Autodesk Inventor part; units mm, degrees
ref_plane "YZ Plane" through (0, 0, 0) normal (1, 0, 0) x (0, 1, 0)
ref_plane "XY Plane" through (0, 0, 0) normal (0, 0, 1) x (1, 0, 0)
sketch "Sketch1" plane through (0, 0, 0) normal (0, 1, 0) x (-1, 0, 0)
  circle A0 centre (0, 0) radius 101.6
  dimension "d0" = 203.2
extrude "Extrusion1" add sketch "Sketch1" along normal mid plane 9.525
sketch "Sketch2" plane through (0, 4.7625, 0) normal (0, 1, 0) x (1, 0, 0)
  circle A0 centre (0, 0) radius 111.125
  dimension "d3" = 222.25
extrude "Extrusion2" add sketch "Sketch2" along normal blind 6.35
mirror "Mirror1" about plane through (0, 0, 0) normal (0, 1, 0) of "Extrusion2"
sketch "Sketch4" plane through (0, 11.1125, 0) normal (0, 1, 0) x (1, 0, 0)
  circle A0 centre (0, 23.8125) radius 2.54
  circle A1 centre (-20.6222, 11.9063) radius 2.54
  circle A2 centre (-20.6222, -11.9062) radius 2.54
  circle A3 centre (0, -23.8125) radius 2.54
  circle A4 centre (20.6222, -11.9063) radius 2.54
  circle A5 centre (20.6222, 11.9062) radius 2.54
  point P0 (0, 0)
  dimension "d6" = 5.08
  dimension "d7" = 23.8125
  dimension "d10" = 360
extrude "Extrusion3" cut sketch "Sketch4" against normal through all
sketch "Sketch5" plane through (0, 11.1125, 0) normal (0, 1, 0) x (1, 0, 0)
  circle A0 centre (0, 0) radius 5
  dimension "d14" = 10
extrude "Extrusion4" cut sketch "Sketch5" against normal through all
equation "\"d0\" = innerDiam"
equation "\"d1\" = innerWidth"
equation "\"d3\" = outerDiam"
equation "\"d4\" = outerWidth"
equation "\"d12\" = outerWidth"
equation "\"d15\" = outerWidth"
equation "\"innerDiam\" = 203.2"
equation "\"innerRadius\" = 0.5 * innerDiam"
equation "\"outerDiam\" = 2 * outerRadius"
equation "\"innerWidth\" = 9.525"
equation "\"outerWidth\" = 6.35"
properties part number "WoodPully"
Build history of the part. All positions in model axes, mm. A direction names the side the tool comes from. Round coordinates to 2 decimals unless told otherwise and drop trailing zeros. Write each loop counter-clockwise with the first axis right and the second up, starting at its lowest first coordinate (ties: lowest second). Pieces come first, ordered by that corner, then holes.
1) Band-saw the part on B-B, the plane x = 0. List the corners of the cut face in (y, z) (1 decimal).
2) 3-axis set-ups, long thin cutter, end or side, ignore diameter. For faces 5 (the flat face through (49, 4.762, 90)), 6 (the flat face through (23, 11.112, -2)): which of +Z, -Z, +X, -X, +Y, -Y reach the whole face in a straight line?
3) Drill centre lines: probe 1 along Z at (x, y) = (0, -5.5) (1 decimal); probe 2 along Z at (x, y) = (0, -1); probe 3 along Y at (x, z) = (-58.5, -85). Where is each one in solid material? Low to high.
4) Band-saw the part on D-D, the plane y = -7.75. Give the number of separate pieces and of enclosed holes in the cut face, and give its area (3 significant figures).
5) Mould opens along Y. For faces 1 (the flat face through (-23, -11.112, -2)), 2 (the cylindrical face through (-18.276, 0.156, 12.879)), 3 (the flat face through (-49, -4.762, 90)), 4 (the cylindrical face through (22.025, 0.067, -99.184)) say: +Y half, -Y half, draft (parallel to the pull), parting line (faces both ways), or undercut.
6) Band-saw the part on C-C, the plane x = 28. List the corners of the cut face in (y, z), and give its area (3 significant figures).
7) Band-saw the part on A-A, the plane z = 0. List the corners of the cut face in (x, y) (1 decimal), and give its area (3 significant figures).
8) Pin check, flat tips, straight feed: pin 1 (10 mm diameter, centred on x = 47, y = -1.5, fed in from +Z); pin 2 (3 mm diameter, centred on x = -20.62, z = 11.91, fed in from +Y); pin 3 (5 mm diameter, centred on x = -10, y = 3.5, fed in from -Z); pin 4 (4 mm diameter, centred on y = 0.5, z = -36.5, fed in from -X). Stop position of each tip, or through.
Ans:
1. outline: (-11.1, -111.1) - (-4.8, -111.1) - (-4.8, -101.6) - (4.8, -101.6) - (4.8, -111.1) - (11.1, -111.1) - (11.1, -26.4) - (-11.1, -26.4) - close; (-11.1, -21.3) - (11.1, -21.3) - (11.1, -5) - (-11.1, -5) - close; (-11.1, 5) - (11.1, 5) - (11.1, 21.3) - (-11.1, 21.3) - close; (-11.1, 26.4) - (11.1, 26.4) - (11.1, 111.1) - (4.8, 111.1) - (4.8, 101.6) - (-4.8, 101.6) - (-4.8, 111.1) - (-11.1, 111.1) - close
2. face 5: none
2. face 6: +Z, -Z, +X, -X, +Y
3. probe 1: z = -111.1 to -26.4, -21.3 to -5, 5 to 21.3, 26.4 to 111.1
3. probe 2: z = -101.6 to -26.35, -21.27 to -5, 5 to 21.27, 26.35 to 101.6
3. probe 3: y = -11.11 to -4.76, 4.76 to 11.11
4. separate pieces: 1
4. enclosed holes: 7
4. area: 38,600 mm2
5. face 1: -Y half
5. face 2: draft
5. face 3: undercut
5. face 4: undercut
6. outline: (-11.11, -107.54) - (-4.76, -107.54) - (-4.76, -97.67) - (4.76, -97.67) - (4.76, -107.54) - (11.11, -107.54) - (11.11, 107.54) - (4.76, 107.54) - (4.76, 97.67) - (-4.76, 97.67) - (-4.76, 107.54) - (-11.11, 107.54) - close
6. area: 4,590 mm2
7. outline: (-111.1, -11.1) - (-5, -11.1) - (-5, 11.1) - (-111.1, 11.1) - (-111.1, 4.8) - (-101.6, 4.8) - (-101.6, -4.8) - (-111.1, -4.8) - close; (5, -11.1) - (111.1, -11.1) - (111.1, -4.8) - (101.6, -4.8) - (101.6, 4.8) - (111.1, 4.8) - (111.1, 11.1) - (5, 11.1) - close
7. area: 4,540 mm2
8. pin 1: stops at z = 102.38
8. pin 2: passes through
8. pin 3: stops at z = -110.85
8. pin 4: stops at x = -95.56
